The model under review builds one solid part; all positions refer to its coordinate system, in mm. A direction names the side the tool comes from. Coordinates: 2 decimals unless noted, no trailing zeros. Order: outer loops, then holes, each group sorted by start corner. A loop starts at its lowest first (then second) coordinate and runs counter-clockwise, first axis right, second up. Notation, with made-up numbers: M -2.5,-10 L 45.5,-10 A29 cw 45.5,27 Z; hole C 17,21.25 d11. An arc over 180 degrees is marked long. One line per item, written item: value.
```python
from build123d import *

# Parameters (mm, degrees)
ESBO_O1_W                = 20
ESBO_O1_H                = 3
RESSALTO_EXTRUS_O1_DEPTH = 2


with BuildPart() as part:
    # Esboço1 → Ressalto-extrusão1 (new body)
    with BuildSketch(Plane(origin=(0, 0, 0), x_dir=(1, 0, 0), z_dir=(0, 1, 0))):
        with BuildLine():
            Line((-10, 10), (-11.599758025, 10))
            ThreePointArc((-11.599758025, 10), (-12.23632523, 9.73632523), (-12.5, 9.099758025))
            Line((-12.5, 9.099758025), (-12.5, -9.099758025))
            ThreePointArc((-12.5, -9.099758025), (-12.23632523, -9.73632523), (-11.599758025, -10))
            Line((-11.599758025, -10), (11.599758025, -10))
            ThreePointArc((11.599758025, -10), (12.23632523, -9.73632523), (12.5, -9.099758025))
            Line((12.5, -9.099758025), (12.5, 9.099758025))
            ThreePointArc((12.5, 9.099758025), (12.23632523, 9.73632523), (11.599758025, 10))
            Line((11.599758025, 10), (10, 10))
            Line((10, 10), (10, 7))
            Line((10, 7), (-10, 7))
            Line((-10, 7), (-10, 10))
        make_face()
        with BuildLine():
            Line((-10, 12.099758025), (-10, 10))
            Line((-10, 10), (10, 10))
            Line((10, 10), (10, 12.099758025))
            ThreePointArc((10, 12.099758025), (9.73632523, 12.73632523), (9.099758025, 13))
            Line((9.099758025, 13), (-9.099758025, 13))
            ThreePointArc((-9.099758025, 13), (-9.73632523, 12.73632523), (-10, 12.099758025))
        make_face()
        with Locations((0, 8.5)):
            Rectangle(ESBO_O1_W, ESBO_O1_H)
    extrude(amount=RESSALTO_EXTRUS_O1_DEPTH)


solid = part.part
```
(1) Tool access review of faces 1 (the flat face through (-12.5, 1, 0)), 2 (the flat face through (11, 1, -10)), 3 (the flat face through (-11, 1, -10)): name each direction out of +Z, -Z, +X, -X, +Y, -Y from which nothing blocks a thin tool from reaching the whole face with its end or side.
Geometry results:
face 1: +Z, -Z, -X, +Y, -Y
face 2: -Z, +X, +Y, -Y
face 3: -Z, -X, +Y, -Y
(2) We need section A-A, the plane y = 1.2. State the section outline as (x, z) points.
Geometry results:
outline: M -12.5,-9.1 A0.9 ccw -11.6,-10 L -10,-10 L -10,-12.1 A0.9 ccw -9.1,-13 L 9.1,-13 A0.9 ccw 10,-12.1 L 10,-10 L 11.6,-10 A0.9 ccw 12.5,-9.1 L 12.5,9.1 A0.9 ccw 11.6,10 L -11.6,10 A0.9 ccw -12.5,9.1 Z
(3) For L1, parallel to Z at x = 10.75, y = 0.8; L2, parallel to Z at x = 9.25, y = 1.95, list the stretches that pass through material, from the lowest coordinate up.
Geometry results:
L1: z = -10 to 10
L2: z = -12.99 to 10
(4) Insertion check: pin 1 Ø0.5 at (x, y) = (10.5, 1) entering from -Z; pin 2 Ø0.6 at (y, z) = (0.5, -10.5) entering from -X; pin 3 Ø1 at (y, z) = (1.5, -11) entering from +X. Each pin has a flat end and moves straight along its axis. Give the tip position at first contact, or say it passes through.
Geometry results:
pin 1: stops at z = -10
pin 2: stops at x = -10
pin 3: stops at x = 10
